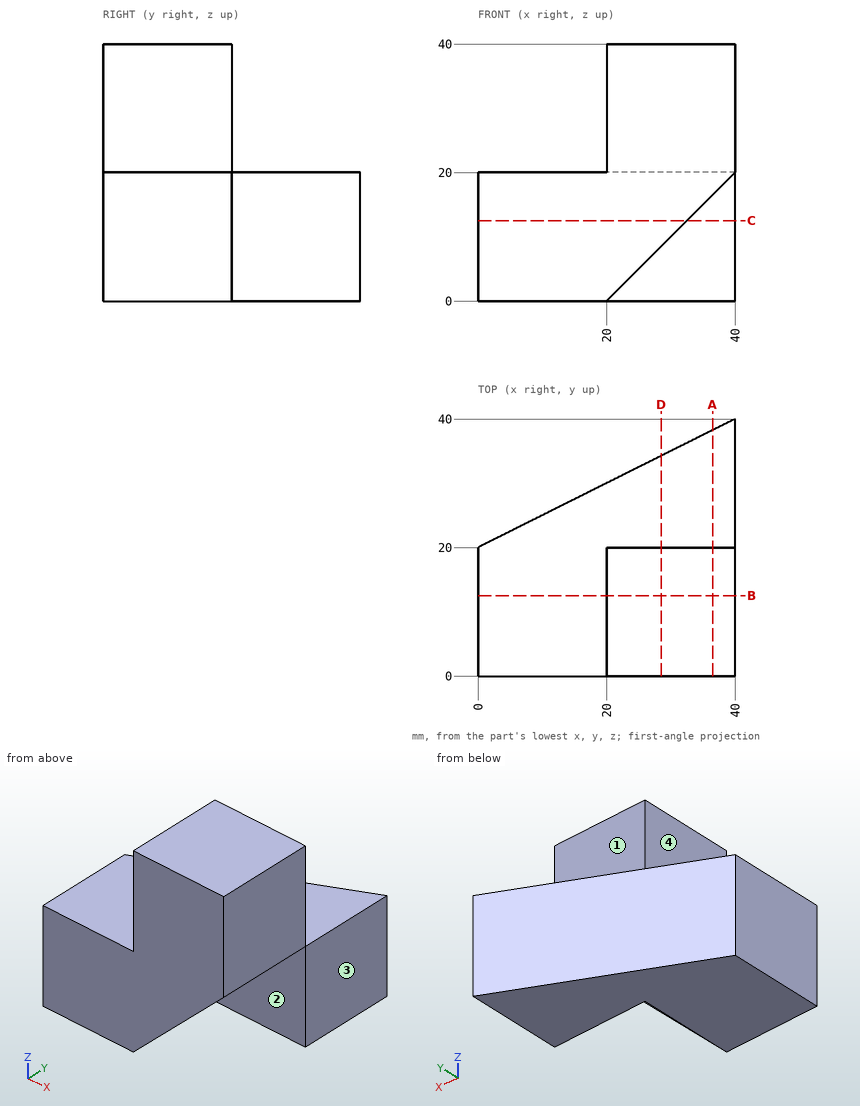
Source: three-view drawing plus pictorial views. Frame: mm from the lowest corner of the part. A direction names the side the tool comes from. Give positions to 0.01 mm unless a question says otherwise; leave off trailing zeros. Write each loop counter-clockwise with the first axis right and the second up, starting at its lowest first coordinate (ties: lowest second). Pieces come first, ordered by that corner, then holes. Notation, with made-up numbers: (79, 65) - (107, 65) arc R9 ccw to (107, 69) - close; hole circle Ø10 at (68.5, -28). An arc over 180 degrees is marked (long way). Write item = value, one per line. Start each with the question number.
1. Section query A-A, the plane x = 36.5. Output: boundary loops of the cut face in (y, z), then the cut area to 3 significant figures.
2. First-contact query: pin 1 Ø10 at (x, z) = (29.5, 31) entering from +Y; pin 2 Ø12 at (x, y) = (32.5, 29.5) entering from +Z; pin 3 Ø12 at (x, z) = (33.5, 18.5) entering from +Y. Flat tips, straight axial feed; report the tip coordinate or a pass-through.
3. Section query B-B, the plane y = 12.5. Output: boundary loops of the cut face in (x, z), then the cut area to 3 significant figures.
4. Access query for the marked faces 1, 2, 3 and 4. Directions: +Z, -Z, +X, -X, +Y, -Y. A direction counts if a zero-diameter tool reaches every point of the face in a straight line with its end or side. Return the directions, or none.
5. Ray query, L1, parallel to X at y = 18, z = 22; L2, parallel to Y at x = 27, z = 37.5. Return the intervals inside material, ascending.
6. Section query D-D, the plane x = 28.5. Output: boundary loops of the cut face in (y, z).
7. Section query C-C, the plane z = 12.5. Output: boundary loops of the cut face in (x, y), then the cut area to 3 significant figures.
Check sheet entries:
q1.outline = (0, 16.5) - (20, 16.5) - (20, 0) - (38.25, 0) - (38.25, 20) - (20, 20) - (20, 40) - (0, 40) - close
q1.area = 835 mm2
q2.pin_1 = 20
q2.pin_2 = 20
q2.pin_3 = 39.75
q3.outline = (0, 0) - (20, 0) - (40, 20) - (40, 40) - (20, 40) - (20, 20) - (0, 20) - close
q3.area = 1,000 mm2
q4.face_1 = +Z, +X, -X, +Y
q4.face_2 = -Z, +X, -Y
q4.face_3 = +Z, -Z, +X, +Y, -Y
q4.face_4 = +Z, -X, +Y, -Y
q5.L1 = 20 to 40
q5.L2 = 0 to 20
q6.outline = (0, 8.5) - (20, 8.5) - (20, 0) - (34.25, 0) - (34.25, 20) - (20, 20) - (20, 40) - (0, 40) - close
q7.outline = (0, 0) - (32.5, 0) - (32.5, 20) - (40, 20) - (40, 40) - (0, 20) - close
q7.area = 1,050 mm2
